Design review of the part built by this model. Coordinates are the model's own, in mm. A direction names the side the tool comes from. Coordinates: 2 decimals unless noted, no trailing zeros. Loops run counter-clockwise (first coordinate to the right, second up) from the corner with the lowest first, then second, coordinate; pieces in that order, holes last. Notation, with made-up numbers: (82.25, -40) -> (132.25, -40) arc R19 cw to (132.25, -24) -> close; hole circle Ø3 at (12.5, 85). An arc over 180 degrees is marked (long way). Answer as a JSON object with one key per item and string values.
Autodesk Fusion 360 part; units mm, degrees
sketch "Sketch1" plane through (0, 0, 0) normal (0, 0, 1) x (1, 0, 0)
  circle A0 centre (0, 0) radius 8.5
  circle A1 centre (0, 0) radius 22.5
  circle A2 centre (0, 0) radius 38
  dimension "d1" = 45
  dimension "d2" = 17
  dimension "d3" = 76
extrude "Extrude1" add sketch "Sketch1" along normal blind 20 contours A1
sketch "Sketch2" plane through (0, 0, 0) normal (0, 0, 1) x (1, 0, 0)
  circle A0 centre (0.2654, -30.1553) radius 2.5
  dimension "d8" = 5
extrude "Extrude4" add sketch "Sketch1" along normal blind 20 contours A1 | A2
extrude "Extrude5" cut sketch "Sketch2" along normal blind 6.312
pattern_circular "C-Pattern2" count 3 over 360 about axis through (0, 0, 20) along (0, 0, 1) of "Extrude5"
1) Add section C-C, the plane z = 18. Give the boundary of the cut face in (x, y), and give its area (3 significant figures).
Completed:
{"outline": "circle Ø76 at (0, 0); hole circle Ø17 at (0, 0)", "area": "4,310 mm²"}
2) Add section D-D, the plane z = 4.25. Give the boundary of the cut face in (x, y), and give its area (3 significant figures).
Completed:
{"outline": "circle Ø76 at (0, 0); hole circle Ø5 at (-26.25, 14.85); hole circle Ø17 at (0, 0); hole circle Ø5 at (0.27, -30.16); hole circle Ø5 at (25.98, 15.31)", "area": "4,250 mm²"}
3) For faces 4 (the flat face through (0, -30, 6.312)), 5 (the flat face through (-1, 9, 20)), list the 3-axis set-ups (+Z, -Z, +X, -X, +Y, -Y) from which the entire face can be reached by the end or side of a thin tool; tool diameter is ignored.
Completed:
{"face 4": "-Z", "face 5": "+Z, +X, -X, +Y, -Y"}
4) Clearance check with flat-ended pins moving along their axes: pin 1 Ø2.5 at (x, y) = (26, 16) entering from -Z; pin 2 Ø5 at (x, y) = (-21.5, 16) entering from -Z; pin 3 Ø5 at (x, z) = (26, 2) entering from +Y; pin 4 Ø5 at (y, z) = (19.5, 15) entering from -X. State where each tip first meets the part, or that it passes through.
Completed:
{"pin 1": "z = 6.31", "pin 2": "z = 0", "pin 3": "y = 29.86", "pin 4": "x = -33.99"}
5) Add section B-B, the plane x = 0. Give the boundary of the cut face in (y, z).
Completed:
{"outline": "(-38, 0) -> (-32.64, 0) -> (-32.64, 6.31) -> (-27.67, 6.31) -> (-27.67, 0) -> (-8.5, 0) -> (-8.5, 20) -> (-38, 20) -> close; (8.5, 0) -> (38, 0) -> (38, 20) -> (8.5, 20) -> close"}
6) The part is to be moulded in two halves that separate along Y. For faces 1 (the cylindrical face through (17.535, 33.713, 9.86)), 2 (the flat face through (-9, 1, 0)), 3 (the cylindrical face through (-23.863, 14.097, 3.112)), say which applies: pulls with the +Y half, pulls with the -Y half, needs draft (parallel to the pull), parting line crosses it, or undercut.
Completed:
{"face 1": "parting line crosses it", "face 2": "needs draft", "face 3": "undercut"}
7) Add section A-A, the plane y = 0. Give the boundary of the cut face in (x, z).
Completed:
{"outline": "(-38, 0) -> (-8.5, 0) -> (-8.5, 20) -> (-38, 20) -> close; (8.5, 0) -> (38, 0) -> (38, 20) -> (8.5, 20) -> close"}
8) Wall thickness on probe 1 along Y at (x, z) = (0, 10.5); probe 2 along X at (y, z) = (-2.5, 2.75); probe 3 along Y at (x, z) = (5.5, 1): over which ranges is each line inside the solid? List them lowest first.
Completed:
{"probe 1": "-38 to -8.5, 8.5 to 38", "probe 2": "-37.92 to -8.12, 8.12 to 37.92", "probe 3": "-37.6 to -6.48, 6.48 to 37.6"}
